```python
from build123d import *

# Parameters (mm, degrees)
SKETCH006_W     = 48
SKETCH006_H     = 28
PAD002_DEPTH    = 4
SKETCH007_W     = 48
SKETCH007_H     = 28
SKETCH007_W_2   = 45
SKETCH007_H_2   = 24
SKETCH007_W_3   = 41.5
SKETCH007_H_3   = 20.5
POCKET004_DEPTH = 1
PAD003_DEPTH    = 1
SKETCH009_R     = 1.1
POCKET005_DEPTH = 4.001
SKETCH010_R     = 2
POCKET006_DEPTH = 2
SKETCH011_W     = 1.5
SKETCH011_H     = 9
SKETCH011_H_2   = 10
PAD004_DEPTH    = 2.6
FILLET002_R     = 1
FILLET003_R     = 1
FILLET004_R     = 0.6


with BuildPart() as part:
    # Sketch006 → Pad002 (new body)
    with BuildSketch(Plane.XY):
        Rectangle(SKETCH006_W, SKETCH006_H)
    extrude(amount=PAD002_DEPTH)

    # Sketch007 (on Face6 of Pad002) → Pocket004 (cut)
    with BuildSketch(Plane.XY.offset(4)):
        Rectangle(SKETCH007_W, SKETCH007_H)
        Rectangle(SKETCH007_W_2, SKETCH007_H_2, mode=Mode.SUBTRACT)
        Rectangle(SKETCH007_W_3, SKETCH007_H_3)
    extrude(amount=-POCKET004_DEPTH, mode=Mode.SUBTRACT)

    # Sketch008 (on Face16 of Pocket004) → Pad003 (join)
    with BuildSketch(Plane.XY.offset(3)):
        with BuildLine():
            Line((5.25, -10.25), (5.25, -8))
            ThreePointArc((10.25, -8), (7.75, -5.5), (5.25, -8))
            Line((10.25, -10.25), (10.25, -8))
            Line((5.25, -10.25), (10.25, -10.25))
        make_face()
        with BuildLine():
            Line((-20.75, 10.25), (-20.75, 5.25))
            Line((-20.75, 5.25), (-16.5, 5.25))
            ThreePointArc((-16.5, 5.25), (-14.732233, 5.982233), (-14, 7.75))
            Line((-14, 7.75), (-14, 10.25))
            Line((-14, 10.25), (-20.75, 10.25))
        make_face()
    extrude(amount=PAD003_DEPTH)

    # Sketch009 (on Face11 of Pad003) → Pocket005 (cut, through all)
    with BuildSketch(Plane.XY.offset(4)):
        with Locations((-16.5, 7.75)):
            Circle(SKETCH009_R)
        with Locations((7.75, -8)):
            Circle(SKETCH009_R)
    extrude(amount=-POCKET005_DEPTH, mode=Mode.SUBTRACT)

    # Sketch010 (on Face2 of Pocket005) → Pocket006 (cut)
    with BuildSketch(Plane(origin=(0, 0, 0), x_dir=(1, 0, 0), z_dir=(0, 0, -1))):
        with Locations((-16.5, -7.75)):
            Circle(SKETCH010_R)
        with Locations((7.75, 8)):
            Circle(SKETCH010_R)
    extrude(amount=-POCKET006_DEPTH, mode=Mode.SUBTRACT)

    # Sketch011 (on Face4 of Pocket006) → Pad004 (join)
    with BuildSketch(Plane.XY.offset(3)):
        with Locations((-23.25, -0.5)):
            Rectangle(SKETCH011_W, SKETCH011_H)
        with Locations((23.25, 0.495)):
            Rectangle(SKETCH011_W, SKETCH011_H_2)
    extrude(amount=PAD004_DEPTH)

    # Fillet002
    fillet002_edges = [part.edges().sort_by_distance(p)[0] for p in [
        (0, -14, 0),
        (-24, 0, 0),
        (-24, -14, 1.5),
        (-24, 14, 1.5),
        (0, 14, 0),
        (24, 0, 0),
        (24, -14, 1.5),
        (24, 14, 1.5),
    ]]
    fillet(fillet002_edges, radius=FILLET002_R)

    # Fillet003
    fillet003_edges = [part.edges().sort_by_distance(p)[0] for p in [
        (5.25, -10.25, 3.5),
        (10.25, -10.25, 3.5),
        (-14, 10.25, 3.5),
        (-20.75, 5.25, 3.5),
        (-20.75, -10.25, 3.5),
        (20.75, 10.25, 3.5),
        (20.75, -10.25, 3.5),
    ]]
    fillet(fillet003_edges, radius=FILLET003_R)

    # Fillet004
    fillet004_edges = [part.edges().sort_by_distance(p)[0] for p in [
        (22.5, 12, 3.5),
        (-22.5, -12, 3.5),
        (-22.5, 12, 3.5),
        (22.5, -12, 3.5),
    ]]
    fillet(fillet004_edges, radius=FILLET004_R)


solid = part.part
```
Check sheet for the modelled part. Datum: model origin and axes. Units: mm. A direction names the side the tool comes from. Coordinates: 2 decimals unless noted, no trailing zeros. Write each loop counter-clockwise with the first axis right and the second up, starting at its lowest first coordinate (ties: lowest second). Pieces come first, ordered by that corner, then holes. Notation, with made-up numbers: M 77.25,79 L 99.25,79 A13 ccw 99.25,92 Z; hole C -20.5,49.25 d6. An arc over 180 degrees is marked long. Write item = value, one per line. Start each with the question number.
1. Thickness scan on probe 1 along Y at (x, z) = (7.75, 3.05); probe 2 along Y at (x, z) = (-16.5, 2.85); probe 3 along Y at (x, z) = (-11, 3.7). Record the ranges inside material, lowest first.
2. Sectioned sample at D-D (x = 2.5). Record the cut outline in (y, z).
3. Go/stop test with flat-tipped pins: pin 1 (0.8 mm diameter, centred on x = 23.5, z = 4, fed in from +Y) (3 decimals); pin 2 (0.5 mm diameter, centred on x = -4, z = 3.5, fed in from +Y); pin 3 (0.8 mm diameter, centred on x = 3, z = 3.5, fed in from -Y). Record where each tip stops, or that it passes through.
4. Mould release check, pull along Y, two halves, no side actions. Record for faces 6 (the cylindrical face through (10.535, -9.949, 3.507)), 7 (the cylindrical face through (23.699, 13.715, 2.014)), 8 (the cylindrical face through (4.949, -9.965, 3.507)), 9 (the flat face through (7, -6, 4)): pulls with the +Y half, pulls with the -Y half, needs draft (parallel to the pull), parting line crosses it, or undercut.
5. Sectioned sample at C-C (z = 4.6). Record the cut outline in (x, y) (3 decimals), then the cut area to 3 significant figures.
6. Sectioned sample at A-A (x = 7.75). Record the cut outline in (y, z), then the cut area to 3 significant figures.
7. Sectioned sample at B-B (y = 2.75). Record the cut outline in (x, z).
8. Tool access check on faces 1 (the flat face through (9, -7, 2)), 2 (the flat face through (-22.5, 7.6, 3.5)), 3 (the cylindrical face through (20.449, 9.965, 3.493)), 4 (the flat face through (22.5, -8, 3.5)), 5 (the flat face through (-22.5, -1, 5)). Record the directions out of +Z, -Z, +X, -X, +Y, -Y that give a thin tool (end or side, any length) a straight path to the whole face; none if there is none.
The answers:
q1.probe_1 = -12 to -9.1, -6.9 to -5.5, 10.25 to 12
q1.probe_2 = -14 to 6.65, 8.85 to 14
q1.probe_3 = -12 to -10.25, 10.25 to 12
q2.outline = M -14,1 A1 ccw -13,0 L 13,0 A1 ccw 14,1 L 14,3 L 12,3 L 12,4 L 10.25,4 L 10.25,3 L -10.25,3 L -10.25,4 L -12,4 L -12,3 L -14,3 Z
q3.pin_1 = 5.495
q3.pin_2 = 12
q3.pin_3 = -12
q4.face_6 = undercut
q4.face_7 = pulls with the +Y half
q4.face_8 = undercut
q4.face_9 = needs draft
q5.outline = M -24,-5 L -22.5,-5 L -22.5,4 L -24,4 Z; M 22.5,-4.505 L 24,-4.505 L 24,5.495 L 22.5,5.495 Z
q5.area = 28.5 mm²
q6.outline = M -14,1 A1 ccw -13,0 L -10,0 L -10,2 L -9.1,2 L -9.1,4 L -12,4 L -12,3 L -14,3 Z; M -6.9,2 L -6,2 L -6,0 L 13,0 A1 ccw 14,1 L 14,3 L 12,3 L 12,4 L 10.25,4 L 10.25,3 L -5.5,3 L -5.5,4 L -6.9,4 Z
q6.area = 79.4 mm²
q7.outline = M -24,1 A1 ccw -23,0 L 23,0 A1 ccw 24,1 L 24,5.6 L 22.5,5.6 L 22.5,4 L 20.75,4 L 20.75,3 L -20.75,3 L -20.75,4 L -22.5,4 L -22.5,5.6 L -24,5.6 Z
q8.face_1 = -Z
q8.face_2 = +Z, -X, +Y
q8.face_3 = +Z
q8.face_4 = +Z, +X, -Y
q8.face_5 = +Z, +Y, -Y
